Can you work these out from the model? Positions are in its coordinate system, mm. Coordinates: 2 decimals unless noted, no trailing zeros. Order: outer loops, then holes, each group sorted by start corner. A loop starts at its lowest first (then second) coordinate and runs counter-clockwise, first axis right, second up.
```python
from build123d import *

# Parameters (mm, degrees)
SKETCH1_W          = 401
SKETCH1_H          = 320
EXTRUDE1_DEPTH     = 8
SKETCH2_W          = 401
SKETCH2_H          = 320
SKETCH2_W_2        = 384.8
SKETCH2_H_2        = 303.8
CUT_EXTRUDE1_DEPTH = 6
SKETCH3_W          = 374.8
SKETCH3_H          = 293.8
CUT_EXTRUDE2_DEPTH = 5.5
FILLET1_R          = 5
SKETCH4_R          = 1.25
CUT_EXTRUDE3_DEPTH = 425.304619348


with BuildPart() as part:
    # Sketch1 → Extrude1 (new body)
    with BuildSketch(Plane(origin=(0, 0, 0), x_dir=(1, 0, 0), z_dir=(0, 1, 0))):
        Rectangle(SKETCH1_W, SKETCH1_H)
    extrude(amount=EXTRUDE1_DEPTH)

    # Sketch2 → Cut-Extrude1 (cut)
    with BuildSketch(Plane(origin=(0, 8, 0), x_dir=(1, 0, 0), z_dir=(0, 1, 0))):
        Rectangle(SKETCH2_W, SKETCH2_H)
        Rectangle(SKETCH2_W_2, SKETCH2_H_2, mode=Mode.SUBTRACT)
    extrude(amount=-CUT_EXTRUDE1_DEPTH, mode=Mode.SUBTRACT)

    # Sketch3 → Cut-Extrude2 (cut)
    with BuildSketch(Plane(origin=(0, 8, 0), x_dir=(1, 0, 0), z_dir=(0, 1, 0))):
        Rectangle(SKETCH3_W, SKETCH3_H)
    extrude(amount=-CUT_EXTRUDE2_DEPTH, mode=Mode.SUBTRACT)

    # Fillet1
    fillet1_edges = [part.edges().sort_by_distance(p)[0] for p in [
        (192.4, 5, 151.9),
        (-192.4, 5, 151.9),
        (-192.4, 5, -151.9),
        (192.4, 5, -151.9),
        (-187.4, 5.25, 146.9),
        (-187.4, 5.25, -146.9),
        (187.4, 5.25, -146.9),
        (187.4, 5.25, 146.9),
    ]]
    fillet(fillet1_edges, radius=FILLET1_R)

    # Sketch4 → Cut-Extrude3 (cut, through all)
    with BuildSketch(Plane.ZY.offset(192.4)):
        with Locations(Location((-101.9, 5, 0), (0, 0, 180))):
            Circle(SKETCH4_R)
        with Locations(Location((101.9, 5, 0), (0, 0, 180))):
            Circle(SKETCH4_R)
    extrude(amount=-CUT_EXTRUDE3_DEPTH, mode=Mode.SUBTRACT)


solid = part.part
```
1. Thinking about a two-plate mould opening in Z: for faces 1 (the flat face through (-3, 0, -2)), 2 (the flat face through (-3, 2.5, -2)), which applies, pulls with the +Z half, pulls with the -Z half, needs draft (parallel to the pull), parting line crosses it, or undercut?
Completed:
face 1: needs draft
face 2: undercut
2. Imagine slicing it at C-C on x = -167. Please give me the cut outline in (y, z).
Completed:
outline: (0, -160) - (2, -160) - (2, -151.9) - (8, -151.9) - (8, -146.9) - (2.5, -146.9) - (2.5, 146.9) - (8, 146.9) - (8, 151.9) - (2, 151.9) - (2, 160) - (0, 160) - close
3. Imagine slicing it at B-B on z = -72. Please give me the cut outline in (x, y), then the cut area to 3 significant figures.
Completed:
outline: (-200.5, 0) - (200.5, 0) - (200.5, 2) - (192.4, 2) - (192.4, 8) - (187.4, 8) - (187.4, 2.5) - (-187.4, 2.5) - (-187.4, 8) - (-192.4, 8) - (-192.4, 2) - (-200.5, 2) - close
area: 1,050 mm2
4. Please list where these lines run through material, in increasing order: probe 1 along Z at (x, y) = (-181, 3); probe 2 along X at (y, z) = (5.25, -140.5); probe 3 along Y at (x, z) = (190.05, -101.9).
Completed:
probe 1: z = -151.9 to -146.9, 146.9 to 151.9
probe 2: x = -192.4 to -187.4, 187.4 to 192.4
probe 3: y = 0 to 3.75, 6.25 to 8
5. I'm going to push flat-ended pins straight in: pin 1 (2 mm diameter, centred on x = -109.5, y = 6, fed in from +Z); pin 2 (3 mm diameter, centred on y = 5, z = 101.9, fed in from +X); pin 3 (8 mm diameter, centred on x = -47.5, z = -35.5, fed in from -Y); pin 4 (4 mm diameter, centred on y = 5, z = -101.9, fed in from -X). Where does each tip first touch, or does it pass through?
Completed:
pin 1: stops at z = 151.9
pin 2: stops at x = 192.4
pin 3: stops at y = 0
pin 4: stops at x = -192.4
6. Imagine slicing it at A-A on y = 5. Give the number of separate pieces and of enclosed holes in the cut face, then the cut area to 3 significant figures.
Completed:
separate pieces: 4
enclosed holes: 0
area: 6,740 mm2
